Autodesk Inventor part; units mm, degrees
ref_plane "YZ Plane" through (0, 0, 0) normal (1, 0, 0) x (0, 1, 0)
ref_plane "XZ Plane" through (0, 0, 0) normal (0, 1, 0) x (-1, 0, 0)
ref_plane "XY Plane" through (0, 0, 0) normal (0, 0, 1) x (1, 0, 0)
sketch "Sketch1" plane through (0, 0, 0) normal (0, 1, 0) x (-1, 0, 0)
  line L0 (25.4, -30.48) -> (43.18, -50.8)
  line L1 (25.4, -96.52) -> (43.18, -76.2)
  line L2 (3.81, 0) -> (0, -3.81)
  line L3 (0, -123.19) -> (3.81, -127)
  line L4 (25.4, -123.19) -> (21.59, -127)
  line L5 (25.4, -3.81) -> (21.59, 0)
  line L6 (72.39, -50.8) -> (76.2, -54.61)
  line L7 (76.2, -72.39) -> (72.39, -76.2)
  line L8 (25.4, -3.81) -> (25.4, -30.48)
  line L9 (43.18, -50.8) -> (72.39, -50.8)
  line L10 (76.2, -54.61) -> (76.2, -72.39)
  line L11 (72.39, -76.2) -> (43.18, -76.2)
  line L12 (25.4, -96.52) -> (25.4, -123.19)
  line L13 (21.59, -127) -> (3.81, -127)
  line L14 (0, -123.19) -> (0, -3.81)
  line L15 (3.81, 0) -> (21.59, 0)
  circle A0 centre (12.7, -12.7) radius 2.54
  circle A1 centre (12.7, -38.1) radius 2.54
  circle A2 centre (12.7, -63.5) radius 2.54
  circle A3 centre (12.7, -88.9) radius 2.54
  circle A4 centre (12.7, -114.3) radius 2.54
  circle A5 centre (63.5, -63.5) radius 2.54
  circle A6 centre (38.1, -63.5) radius 2.54
  circle A7 centre (22.86, -53.34) radius 2.54
  circle A8 centre (22.86, -73.66) radius 2.54
  point P0 (0, 0)
extrude "Extrusion1" add sketch "Sketch1" along normal blind 2.54
properties part number "1in tbracket for alu extrusions" material "Steel, Alloy"
Could you check a few things on this model? Use its own coordinates, in mm. A direction names the side the tool comes from. Coordinates: 2 decimals unless noted, no trailing zeros. Write each loop counter-clockwise with the first axis right and the second up, starting at its lowest first coordinate (ties: lowest second). Pieces come first, ordered by that corner, then holes. Notation, with made-up numbers: (88, 35) - (102, 35) arc R33 cw to (102, 66) - close; hole circle Ø11 at (-30, -14). An arc over 180 degrees is marked (long way). Put each result on its own line as item: value. Start each with the question number.
Q1. I want a section at D-D on y = 0.55. Count the separate pieces of the cut face and the enclosed holes in it, plus the area to 3 significant figures.
Q2. I'm going to push flat-ended pins straight in: P1, Ø1.3, axis at y = 1.5, z = -107, coming from the -X side; P2, Ø1.5, axis at x = -41, y = 1.5, coming from the +Z side; P3, Ø0.8, axis at x = -61.5, y = 2, coming from the -Z side. Where does each tip first touch, or does it pass through?
Q3. I want a section at B-B on z = -53.34. Write out the boundary of the cut face in (x, y), plus the area to 3 significant figures.
Q4. Thinking about a two-plate mould opening in Z: for faces 4 (the cylindrical face through (-12.15, 1.25, -61.02)), 5 (the flat face through (-34.17, 1.25, -86.5)), 6 (the flat face through (-25.4, 1, -110)), which applies, pulls with the +Z half, pulls with the -Z half, needs draft (parallel to the pull), parting line crosses it, or undercut?
Q5. I want a section at A-A on x = -63.5. Write out the boundary of the cut face in (y, z), plus the area to 3 significant figures.
Q6. Please list where these lines run through material, in increasing order: L1, parallel to Z at x = -12.7, y = 0.85; L2, parallel to X at y = 1.65, z = -25; L3, parallel to X at y = 1.4, z = -115.5.
Q7. I want a section at C-C on x = -12.7. Write out the boundary of the cut face in (y, z).
Q8. Which directions (+Z, -Z, +X, -X, +Y, -Y) give clear straight access to the entire face, cutting with the end or side of a thin tool? Please do faces 1 (the flat face through (-58, 1, -50.8)), 2 (the flat face through (-58, 1, -76.2)), 3 (the cylindrical face through (-36.084, 1.252, -61.954)).
Checks:
1. separate pieces: 1
1. enclosed holes: 9
1. area: 4,650 mm²
2. P1: x = -25.4
2. P2: z = -47.45
2. P3: z = -76.2
3. outline: (-74.93, 0) - (-25.4, 0) - (-25.4, 2.54) - (-74.93, 2.54) - close; (-20.32, 0) - (0, 0) - (0, 2.54) - (-20.32, 2.54) - close
3. area: 177 mm²
4. face 4: undercut
4. face 5: pulls with the -Z half
4. face 6: needs draft
5. outline: (0, -76.2) - (2.54, -76.2) - (2.54, -66.04) - (0, -66.04) - close; (0, -60.96) - (2.54, -60.96) - (2.54, -50.8) - (0, -50.8) - close
5. area: 51.6 mm²
6. L1: -127 to -116.84, -111.76 to -91.44, -86.36 to -66.04, -60.96 to -40.64, -35.56 to -15.24, -10.16 to 0
6. L2: -25.4 to 0
6. L3: -25.4 to -14.94, -10.46 to 0
7. outline: (0, -127) - (2.54, -127) - (2.54, -116.84) - (0, -116.84) - close; (0, -111.76) - (2.54, -111.76) - (2.54, -91.44) - (0, -91.44) - close; (0, -86.36) - (2.54, -86.36) - (2.54, -66.04) - (0, -66.04) - close; (0, -60.96) - (2.54, -60.96) - (2.54, -40.64) - (0, -40.64) - close; (0, -35.56) - (2.54, -35.56) - (2.54, -15.24) - (0, -15.24) - close; (0, -10.16) - (2.54, -10.16) - (2.54, 0) - (0, 0) - close
8. face 1: +Z, -X, +Y, -Y
8. face 2: -Z, -X, +Y, -Y
8. face 3: +Y, -Y
